```python
from build123d import *

# Parameters (mm, degrees)
F0_W     = 30
F0_H     = 32
F1_DEPTH = 5
F2_W     = 30
F2_H     = 5
F3_DEPTH = 20
F4_R     = 3
F5_DEPTH = 25
F6_R     = 2.5
F7_DEPTH = 25


with BuildPart() as f1:
    # F0 (on Front) → F1 (new body)
    with BuildSketch(Plane.XZ):
        with Locations((15, 16)):
            Rectangle(F0_W, F0_H)
    extrude(amount=F1_DEPTH)

    # F2 (on face) → F3 (join)
    with BuildSketch(Plane(origin=(0, 0, 0), x_dir=(-1, 0, 0), z_dir=(0, 1, 0))):
        with Locations((-15, 2.5)):
            Rectangle(F2_W, F2_H)
    extrude(amount=F3_DEPTH)

    # F4 (on face) → F5 (cut)
    with BuildSketch(Plane.XY.offset(5)):
        with Locations((23, 10)):
            Circle(F4_R)
        with Locations((7, 10)):
            Circle(F4_R)
    extrude(amount=-F5_DEPTH, mode=Mode.SUBTRACT)

    # F6 (on face) → F7 (cut)
    with BuildSketch(Plane.XZ.offset(5)):
        with Locations((15, 26)):
            Circle(F6_R)
    extrude(amount=-F7_DEPTH, mode=Mode.SUBTRACT)


solid = f1.part
```
Can you work these out from the model? Positions are in its coordinate system, mm. A direction names the side the tool comes from. Coordinates: 2 decimals unless noted, no trailing zeros. Loops run counter-clockwise (first coordinate to the right, second up) from the corner with the lowest first, then second, coordinate; pieces in that order, holes last. Notation, with made-up numbers: M -6,-27 L 10,-27 A29 cw 10,-4 Z; hole C -13.75,49.5 d8. An arc over 180 degrees is marked long. Put each result on its own line as item: value. Start each with the question number.
(1) Imagine slicing it at D-D on x = 23. List the corners of the cut face in (y, z) for me, and give its area (3 significant figures).
(2) We'd pull the mould along X, two halves only. Please class faces 3 (the face through (30, -2, 10)), 4 (the face through (13.16, -2.54, 27.69)), 5 (the face through (15, 20, 3)): +X half, -X half, draft (parallel to the pull), parting line (faces both ways), or undercut.
(3) I need wall thicknesses on probe 1 along Z at (x, y) = (15, -3.3); probe 2 along Z at (x, y) = (5.75, 18.5); probe 3 along Y at (x, z) = (23, 3.1). Which ranges of each line are inside material? Lowest first, please.
(4) Imagine slicing it at A-A on y = 10. List the corners of the cut face in (x, z) for me, and give its area (3 significant figures).
(5) Imagine slicing it at B-B on x = 15. List the corners of the cut face in (y, z) for me, and give its area (3 significant figures).
(6) Imagine slicing it at C-C on z = 26. List the corners of the cut face in (x, y) for me.
(7) Will these pins go through, and if not, where does the flat tip stop? pin 1 Ø12 at (x, z) = (25, 16.5) entering from +Y; pin 2 Ø6 at (x, y) = (8.5, 13.5) entering from +Z.
(8) Which directions (+Z, -Z, +X, -X, +Y, -Y) give clear straight access to the entire face, cutting with the end or side of a thin tool? Please do faces 1 (the face through (15, 7, 0)), 2 (the face through (15, 10, 5)).
Worked answers:
1. outline: M -5,0 L 7,0 L 7,5 L 0,5 L 0,32 L -5,32 Z; M 13,0 L 20,0 L 20,5 L 13,5 Z
1. area: 230 mm2
2. face 3: +X half
2. face 4: undercut
2. face 5: draft
3. probe 1: z = 0 to 23.5, 28.5 to 32
3. probe 2: z = 0 to 5
3. probe 3: y = -5 to 7, 13 to 20
4. outline: M 0,0 L 4,0 L 4,5 L 0,5 Z; M 10,0 L 20,0 L 20,5 L 10,5 Z; M 26,0 L 30,0 L 30,5 L 26,5 Z
4. area: 90.0 mm2
5. outline: M -5,0 L 20,0 L 20,5 L 0,5 L 0,23.5 L -5,23.5 Z; M -5,28.5 L 0,28.5 L 0,32 L -5,32 Z
5. area: 235 mm2
6. outline: M 0,-5 L 12.5,-5 L 12.5,0 L 0,0 Z; M 17.5,-5 L 30,-5 L 30,0 L 17.5,0 Z
7. pin 1: stops at y = 0
7. pin 2: stops at z = 5
8. face 1: -Z, +X, -X, +Y, -Y
8. face 2: +Z, +X, -X, +Y
